from build123d import *

# Parameters (mm, degrees)
EXTRUDE_1_DEPTH       = 1.6
SKETCH_5_R            = 2.6
CUT_EXTRUDE_855_DEPTH = 1
CUT_EXTRUDE_992_REACH = 42.148
SKETCH_7_R            = 1.25
CUT_EXTRUDE_1_REACH   = 42.168
SKETCH_9_W            = 40
SKETCH_9_H            = 4.4


with BuildPart() as part:
    # 草图1 → 凸台-拉伸1 (new body)
    with BuildSketch(Plane(origin=(0, 0, 0), x_dir=(1, 0, 0), z_dir=(0, 1, 0))):
        with BuildLine():
            Line((-30.1, -22.7), (30.1, -22.7))
            ThreePointArc((30.1, -22.7), (32.221320344, -21.821320344), (33.1, -19.7))
            Line((33.1, -19.7), (33.1, 19.7))
            ThreePointArc((33.1, 19.7), (32.221320344, 21.821320344), (30.1, 22.7))
            Line((30.1, 22.7), (-30.1, 22.7))
            ThreePointArc((-30.1, 22.7), (-32.221320344, 21.821320344), (-33.1, 19.7))
            Line((-33.1, 19.7), (-33.1, -19.7))
            ThreePointArc((-33.1, -19.7), (-32.221320344, -21.821320344), (-30.1, -22.7))
        make_face()
    extrude(amount=EXTRUDE_1_DEPTH)

    # 草图5 → Cut-Extrude 855 (cut)
    with BuildSketch(Plane.XZ):
        with Locations(Location((-28, -17.6, 0), (0, 0, 270))):
            Circle(SKETCH_5_R)
        with Locations(Location((28, -17.6, 0), (0, 0, 270))):
            Circle(SKETCH_5_R)
        with Locations(Location((28, 17.4, 0), (0, 0, 270))):
            Circle(SKETCH_5_R)
        with Locations(Location((-28, 17.4, 0), (0, 0, 270))):
            Circle(SKETCH_5_R)
    extrude(amount=-CUT_EXTRUDE_855_DEPTH, mode=Mode.SUBTRACT)

    # 草图7 → Cut-Extrude 992 (cut, up to next)
    with BuildSketch(Plane.XZ.offset(-1), mode=Mode.PRIVATE) as cut_extrude_992_sk1:
        with Locations(Location((-28, -17.6, 0), (0, 0, 270))):
            Circle(SKETCH_7_R)
    cut_extrude_992_tool1 = extrude(cut_extrude_992_sk1.sketch, amount=-CUT_EXTRUDE_992_REACH, mode=Mode.PRIVATE) & part.part
    # 草图7 → Cut-Extrude 992 (cut, up to next)
    with BuildSketch(Plane.XZ.offset(-1), mode=Mode.PRIVATE) as cut_extrude_992_sk2:
        with Locations(Location((28, -17.6, 0), (0, 0, 270))):
            Circle(SKETCH_7_R)
    cut_extrude_992_tool2 = extrude(cut_extrude_992_sk2.sketch, amount=-CUT_EXTRUDE_992_REACH, mode=Mode.PRIVATE) & part.part
    # 草图7 → Cut-Extrude 992 (cut, up to next)
    with BuildSketch(Plane.XZ.offset(-1), mode=Mode.PRIVATE) as cut_extrude_992_sk3:
        with Locations(Location((28, 17.4, 0), (0, 0, 270))):
            Circle(SKETCH_7_R)
    cut_extrude_992_tool3 = extrude(cut_extrude_992_sk3.sketch, amount=-CUT_EXTRUDE_992_REACH, mode=Mode.PRIVATE) & part.part
    # 草图7 → Cut-Extrude 992 (cut, up to next)
    with BuildSketch(Plane.XZ.offset(-1), mode=Mode.PRIVATE) as cut_extrude_992_sk4:
        with Locations(Location((-28, 17.4, 0), (0, 0, 270))):
            Circle(SKETCH_7_R)
    cut_extrude_992_tool4 = extrude(cut_extrude_992_sk4.sketch, amount=-CUT_EXTRUDE_992_REACH, mode=Mode.PRIVATE) & part.part
    add(cut_extrude_992_tool1.solids().sort_by_distance((-28, 1, -17.6))[0], mode=Mode.SUBTRACT)
    add(cut_extrude_992_tool2.solids().sort_by_distance((28, 1, -17.6))[0], mode=Mode.SUBTRACT)
    add(cut_extrude_992_tool3.solids().sort_by_distance((28, 1, 17.4))[0], mode=Mode.SUBTRACT)
    add(cut_extrude_992_tool4.solids().sort_by_distance((-28, 1, 17.4))[0], mode=Mode.SUBTRACT)

    # 草图9 → 切除-拉伸1 (cut, up to next)
    with BuildSketch(Plane(origin=(0, 0, 0), x_dir=(-1, 0, 0), z_dir=(0, -1, 0)), mode=Mode.PRIVATE) as cut_extrude_1_sk1:
        with Locations((-4.1, -18.3)):
            Rectangle(SKETCH_9_W, SKETCH_9_H)
    cut_extrude_1_tool1 = extrude(cut_extrude_1_sk1.sketch, amount=-CUT_EXTRUDE_1_REACH, mode=Mode.PRIVATE) & part.part
    # 草图9 → 切除-拉伸1 (cut, up to next)
    with BuildSketch(Plane(origin=(0, 0, 0), x_dir=(-1, 0, 0), z_dir=(0, -1, 0)), mode=Mode.PRIVATE) as cut_extrude_1_sk2:
        with BuildLine():
            Line((-16.900000063, -8), (-16.900000063, -9.000012563))
            ThreePointArc((-16.900000063, -9.000012563), (-17.613889315, -10.705332368), (-15.905012563, -10))
            Line((-15.905012563, -10), (14.1, -10))
            ThreePointArc((14.1, -10), (15.807106781, -10.707106781), (15.1, -9))
            Line((15.1, -9), (15.1, 7))
            ThreePointArc((15.1, 7), (15.770820393, 8.741619849), (14.105012563, 7.9))
            Line((14.105012563, 7.9), (-15.905012563, 7.9))
            ThreePointArc((-15.905012563, 7.9), (-17.57082037, 8.74161987), (-16.900000063, 7))
            Line((-16.900000063, 7), (-16.900000063, 5.9))
            Line((-16.900000063, 5.9), (-19.900000063, 5.9))
            Line((-19.900000063, 5.9), (-19.900000063, -8))
            Line((-19.900000063, -8), (-16.900000063, -8))
        make_face()
    cut_extrude_1_tool2 = extrude(cut_extrude_1_sk2.sketch, amount=-CUT_EXTRUDE_1_REACH, mode=Mode.PRIVATE) & part.part
    add(cut_extrude_1_tool1.solids().sort_by_distance((4.1, 0, 18.3))[0], mode=Mode.SUBTRACT)
    add(cut_extrude_1_tool2.solids().sort_by_distance((2.069376, 0, 1.046434))[0], mode=Mode.SUBTRACT)


solid = part.part
Geometry: final body of the model. Coordinates: model frame, mm. A direction names the side the tool comes from. Round coordinates to 2 decimals unless told otherwise and drop trailing zeros. Order: outer loops, then holes, each group sorted by start corner. A loop starts at its lowest first (then second) coordinate and runs counter-clockwise, first axis right, second up.
Q1. Mould query, pull axis Z, two halves, no side actions, for faces 1 (the face through (0, 1, 22.7)), 2 (the face through (-15.9, 1, 18)), 3 (the face through (33.1, 1, 0)). Classes: released by +Z, released by -Z, zero draft, split by the parting line, or undercut.
Result sheet:
face 1: released by +Z
face 2: undercut
face 3: zero draft
Q2. Access query for faces 4 (the face through (-32.24, 0.79, 21.8)), 5 (the face through (24.1, 1, 18)), 6 (the face through (-27.9, 0.5, 20)). Directions: +Z, -Z, +X, -X, +Y, -Y. A direction counts if a zero-diameter tool reaches every point of the face in a straight line with its end or side. Return the directions, or none.
Result sheet:
face 4: +Z, -X, +Y, -Y
face 5: +Y, -Y
face 6: -Y
Q3. Material intervals for probe 1 along X at (y, z) = (1.35, -8); probe 2 along Z at (x, y) = (-7.5, 0.95); probe 3 along X at (y, z) = (0.55, -17.6), sorted ascending.
Result sheet:
probe 1: x = -33.1 to -16.1, -14.1 to 15.9, 17.9 to 33.1
probe 2: z = -22.7 to -7.9, 10 to 16.1, 20.5 to 22.7
probe 3: x = -33.1 to -30.6, -25.4 to 25.4, 30.6 to 33.1
Q4. Section C-C, the plane x = -28. Output: boundary loops of the cut face in (y, z).
Result sheet:
outline: (0, -22.7) - (1.6, -22.7) - (1.6, -18.85) - (1, -18.85) - (1, -20.2) - (0, -20.2) - close; (0, -15) - (1, -15) - (1, -16.35) - (1.6, -16.35) - (1.6, 16.15) - (1, 16.15) - (1, 14.8) - (0, 14.8) - close; (0, 20) - (1, 20) - (1, 18.65) - (1.6, 18.65) - (1.6, 22.7) - (0, 22.7) - close
Q5. Section B-B, the plane y = 0.7. Output: boundary loops of the cut face in (x, z), and give its area (3 significant figures).
Result sheet:
outline: (-33.1, -19.7) arc R3 ccw to (-30.1, -22.7) - (30.1, -22.7) arc R3 ccw to (33.1, -19.7) - (33.1, 19.7) arc R3 ccw to (30.1, 22.7) - (-30.1, 22.7) arc R3 ccw to (-33.1, 19.7) - close; hole circle Ø5.2 at (-28, -17.6); hole circle Ø5.2 at (-28, 17.4); hole (-15.9, 16.1) - (24.1, 16.1) - (24.1, 20.5) - (-15.9, 20.5) - close; hole (-15.1, -7) arc R1 ccw (long way) to (-14.11, -7.9) - (15.91, -7.9) arc R1 ccw (long way) to (16.9, -7) - (16.9, -5.9) - (19.9, -5.9) - (19.9, 8) - (16.9, 8) - (16.9, 9) arc R1 ccw (long way) to (15.91, 10) - (-14.1, 10) arc R1 ccw (long way) to (-15.1, 9) - close; hole circle Ø5.2 at (28, -17.6); hole circle Ø5.2 at (28, 17.4)
area: 2,110 mm2
Q6. Pin query (flat end, axial travel): pin 1 (4.5 mm diameter, centred on x = -28, z = -17.6, fed in from -Y); pin 2 (5 mm diameter, centred on x = -17.5, z = -17.5, fed in from -Y); pin 3 (8 mm diameter, centred on x = 11, z = -1, fed in from +Y). Return the tip coordinate at first contact, or that it passes through.
Result sheet:
pin 1: stops at y = 1
pin 2: stops at y = 0
pin 3: passes through
Q7. Section D-D, the plane z = 17.4. Output: boundary loops of the cut face in (x, y), and give its area (3 significant figures).
Result sheet:
outline: (-33.1, 0) - (-30.6, 0) - (-30.6, 1) - (-29.25, 1) - (-29.25, 1.6) - (-33.1, 1.6) - close; (-26.75, 1) - (-25.4, 1) - (-25.4, 0) - (-15.9, 0) - (-15.9, 1.6) - (-26.75, 1.6) - close; (24.1, 0) - (25.4, 0) - (25.4, 1) - (26.75, 1) - (26.75, 1.6) - (24.1, 1.6) - close; (29.25, 1) - (30.6, 1) - (30.6, 0) - (33.1, 0) - (33.1, 1.6) - (29.25, 1.6) - close
area: 28.5 mm2
Q8. Section A-A, the plane z = -17.6. Output: boundary loops of the cut face in (x, y).
Result sheet:
outline: (-33.1, 0) - (-30.6, 0) - (-30.6, 1) - (-29.25, 1) - (-29.25, 1.6) - (-33.1, 1.6) - close; (-26.75, 1) - (-25.4, 1) - (-25.4, 0) - (25.4, 0) - (25.4, 1) - (26.75, 1) - (26.75, 1.6) - (-26.75, 1.6) - close; (29.25, 1) - (30.6, 1) - (30.6, 0) - (33.1, 0) - (33.1, 1.6) - (29.25, 1.6) - close
